from build123d import *

# Parameters (mm, degrees)
F2_S7_R     = 5.66
F2_T8_DEPTH = 10
F3_R        = 0.1
F4_D        = 2.2606
F4_DEPTH    = 6.001


# Not quite as in the source:
# - a fillet or chamfer that OpenCascade refuses, or shapes differently, is made with other operations: its cross-section is extruded or revolved along the edge and cut away or added


with BuildPart() as f1:
    # F0 (on Front) → F1 (revolve)
    with BuildSketch(Plane.XZ):
        Polygon((4.75, 4), (4.75, 0), (5.66, 0), (5.66, 2.7), (6, 2.7), (6, 14.05), (5, 14.05), (5, 15.85), (0, 15.85), (0, 12.954), (1.61, 12.954), (1.61, 4), align=None)
    revolve(axis=Axis((0, 0, 9.925), (0, 0, 1)))

    # F2: chamfer of 0.7 on 3 edges, made by hand

    # F2_s1 → F2_t2 (revolve, cut)
    with BuildSketch(Plane.XZ):
        Polygon((6, 13.35), (5.3, 14.05), (6, 14.05), align=None)
    revolve(axis=Axis((0, 0, 14.05), (0, 0, 1)), mode=Mode.SUBTRACT)


with BuildPart() as f2_tool4:
    # F2_s5 → F2_t6 (revolve)
    with BuildSketch(Plane.XZ):
        Polygon((5.3, 2.7), (6, 3.4), (6, 2.7), align=None)
    revolve(axis=Axis((0, 0, 2.7), (0, 0, 1)))

    # F2_s7 → F2_t8 (cut, symmetric)
    with BuildSketch(Plane.XY.offset(3.1)):
        Circle(F2_S7_R)
    extrude(amount=F2_T8_DEPTH, both=True, mode=Mode.SUBTRACT)


with BuildPart() as f1_1:
    add(f1.part)

    # F2_t3: cut F2_tool4
    add(f2_tool4.part, mode=Mode.SUBTRACT)

    # F2_s9 → F2_t10 (revolve, cut)
    with BuildSketch(Plane.XZ):
        Polygon((5, 15.15), (4.3, 15.85), (5, 15.85), align=None)
    revolve(axis=Axis((0, 0, 15.85), (0, 0, 1)), mode=Mode.SUBTRACT)

    # F3
    f3_edges = [f1_1.edges().sort_by_distance(p)[0] for p in [
        (-5.66, 0, 0),
    ]]
    fillet(f3_edges, radius=F3_R)

    # F4 (through all, one way)
    with BuildSketch(Plane.XZ):
        with Locations((0, 7.239)):
            Circle(F4_D / 2)
    extrude(amount=-F4_DEPTH, mode=Mode.SUBTRACT)


solid = f1_1.part
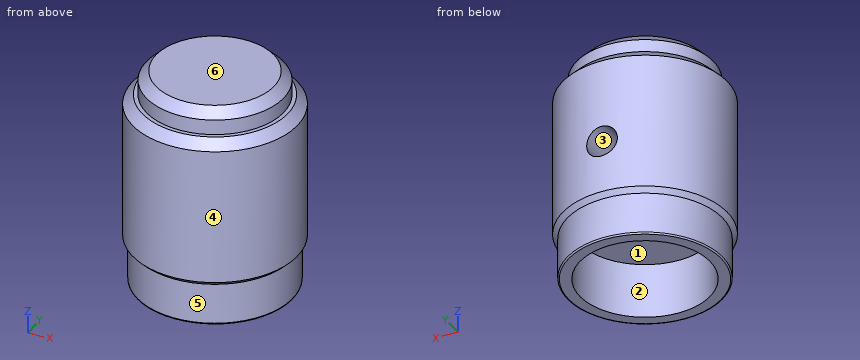
Source: CAD feature listing. Evaluate the final solid. Frame: model axes, mm. Face numbers are marked on the shaded views. A direction names the side the tool comes from. Coordinates: 2 decimals unless noted, no trailing zeros. Order: outer loops, then holes, each group sorted by start corner. A loop starts at its lowest first (then second) coordinate and runs counter-clockwise, first axis right, second up. Notation, with made-up numbers: M -4,13.5 L 33,13.5 A10 ccw 33,23.5 Z; hole C 43,54 d5. An arc over 180 degrees is marked long. Write each question's results on one line, items separated by ' | '. Start each with the question number.
Item 1: Cut plane D-D (z = 7.75). Return loops of the section in (x, y).
Item 2: First-contact query: pin 1 Ø1.6 at (x, y) = (-1, 0.5) entering from -Z; pin 2 Ø1 at (x, z) = (-4.5, 9) entering from +Y; pin 3 Ø3 at (y, z) = (-3, 3) entering from +X. Flat tips, straight axial feed; report the tip coordinate or a pass-through.
Item 3: Set-up query: the marked faces 5 and 6. Return all of +Z, -Z, +X, -X, +Y, -Y with unobstructed straight access to the full face (end or side cutting, diameter ignored); none if empty.
Item 4: Line query: probe 1 along Y at (x, z) = (0, 0.85); probe 2 along Z at (x, y) = (0, 2.7); probe 3 along Y at (x, z) = (0, 8.75). Output: solid intervals per line, ascending.
Item 5: Draft query along Y for the marked faces 1, 2, 3 and 4. Return one class per face: pulls with the +Y half, pulls with the -Y half, needs draft (parallel to the pull), parting line crosses it, or undercut.
Item 6: Cut plane C-C (z = 5.75). Return loops of the section in (x, y).
Item 7: Cut plane B-B (y = 0). Return loops of the section in (x, z).
Checked values:
1) outline: M -1.01,1.26 L -1.01,5.91 A6 ccw long 1.01,5.91 L 1.01,1.26 A1.61 cw long Z
2) pin 1: stops at z = 4 | pin 2: stops at y = 4.47 | pin 3: stops at x = 5.8
3) face 5: -Z | face 6: +Z, +X, -X, +Y, -Y
4) probe 1: y = -5.66 to -4.75, 4.75 to 5.66 | probe 2: z = 4 to 6.11, 8.37 to 15.85 | probe 3: y = -6 to -1.61, 1.61 to 6
5) face 1: undercut | face 2: undercut | face 3: needs draft | face 4: parting line crosses it
6) outline: C 0,0 d12; hole C 0,0 d3.22
7) outline: M -6,3.4 L -5.66,3.06 L -5.66,0.1 A0.1 ccw -5.56,0 L -4.75,0 L -4.75,4 L -1.61,4 L -1.61,12.95 L 1.61,12.95 L 1.61,4 L 4.75,4 L 4.75,0 L 5.56,0 A0.1 ccw 5.66,0.1 L 5.66,3.06 L 6,3.4 L 6,13.35 L 5.3,14.05 L 5,14.05 L 5,15.15 L 4.3,15.85 L -4.3,15.85 L -5,15.15 L -5,14.05 L -5.3,14.05 L -6,13.35 Z
